Read the model definition and answer for the solid it produces. Units are mm, in the model's axes. Face numbers are marked on the shaded views. A direction names the side the tool comes from. Coordinates: 2 decimals unless noted, no trailing zeros. Write each loop counter-clockwise with the first axis right and the second up, starting at its lowest first coordinate (ties: lowest second). Pieces come first, ordered by that corner, then holes.
(1) Which of the six approach directions +Z, -Z, +X, -X, +Y, -Y give full straight-line access (tool end or side, diameter ignored) to the marked faces 4 and 5?
(2) The part is cut by section C-C, the plane z = 0. Determine the outline of the cut face in (x, y), and give its area (3 significant figures).
(3) Straight lines are drawn through the part: line 1 along Z through (x, y) = (4, -2); line 2 along Y through (x, z) = (5.5, 3); line 3 along X through (y, z) = (-7.5, 10). For each, find the intervals that lie inside material, in ascending order.
(4) Determine the mould class of the marked faces 1, 2 and 3 for opening direction Z: pulls with the +Z half, pulls with the -Z half, needs draft (parallel to the pull), parting line crosses it, or undercut.
(5) Given pin 1 (4 mm diameter, centred on x = 5, y = 11, fed in from +Z); pin 2 (2 mm diameter, centred on y = -14.5, z = 3.5, fed in from +X); pin 3 (2 mm diameter, centred on x = 4, z = 14, fed in from -Y); pin 4 (4 mm diameter, centred on y = -16, z = 0, fed in from +X), each flat-ended and moving along its own axis, determine where each tip first touches the part or whether it passes through.
(6) The part is cut by section D-D, the plane x = 20.25. Determine the outline of the cut face in (y, z).
(7) The part is cut by section A-A, the plane z = 16. Determine the outline of the cut face in (x, y).
Autodesk Inventor part; units mm, degrees
ref_plane "YZ Plane" through (0, 0, 0) normal (1, 0, 0) x (0, 1, 0)
ref_plane "XZ Plane" through (0, 0, 0) normal (0, 1, 0) x (-1, 0, 0)
ref_plane "XY Plane" through (0, 0, 0) normal (0, 0, 1) x (1, 0, 0)
sketch "Sketch_1" plane through (0, 0, 0) normal (0, 0, 1) x (1, 0, 0)
  line L0 (24, 0) -> (0, 0)
  line L1 (0, 20) -> (0, 6)
  line L2 (0, 6) -> (24, 6)
  line L3 (24, 6) -> (24, 11)
  line L4 (24, 11) -> (6, 11)
  line L5 (6, 11) -> (6, 20)
  line L6 (6, 20) -> (0, 20)
revolve "Revolution1" add sketch "Sketch_1" angle 360 about axis through (24, 0, 0) along (1, 0, 0)
sketch "Sketch2" plane through (0, 0, 0) normal (-1, 0, 0) x (0, 0, 1)
  point P0 (0, 16)
hole "Hole1" at (0, 16, 0) direction (1, 0, 0) diameter 4.5 depth 6
pattern_linear "Rectangular Pattern1" count 2 spacing 22.6274 along (0, -0.7071, 0.7071) count 2 spacing 22.6274 along (0, -0.7071, -0.7071) of "Hole1"
sketch "Sketch_4" plane through (15, 0, 0) normal (1, 0, 0) x (0, 0, -1)
  line L0 (-7.7782, -7.7782) -> (-3.5355, -3.5355)
  line L1 (-3.5355, -3.5355) -> (-2.3893, -4.6818)
  line L2 (-2.3893, -4.6818) -> (-6.364, -8.6564)
  line L3 (-6.364, -8.6564) -> (-6.364, -9.1924)
  line L4 (-6.364, -9.1924) -> (-7.7782, -7.7782)
  line L5 (-7.7782, -7.7782) -> (-3.5355, -3.5355)
revolve "Revolution2" cut sketch "Sketch_4" angle 360 about axis through (15, -7.7782, 7.7782) along (0, -0.7071, 0.7071)
thread "Thread1"
sketch "Sketch_5" plane through (15, 0, 0) normal (1, 0, 0) x (0, 0, -1)
  line L0 (-7.7782, 7.7782) -> (-3.5355, 3.5355)
  line L1 (-3.5355, 3.5355) -> (-4.6818, 2.3893)
  line L2 (-4.6818, 2.3893) -> (-8.6564, 6.364)
  line L3 (-8.6564, 6.364) -> (-9.1924, 6.364)
  line L4 (-9.1924, 6.364) -> (-7.7782, 7.7782)
  line L5 (-7.7782, 7.7782) -> (-3.5355, 3.5355)
revolve "Revolution3" cut sketch "Sketch_5" angle 360 about axis through (15, 7.7782, 7.7782) along (0, 0.7071, 0.7071)
thread "Thread2"
properties part number "STHRBN12_ss"
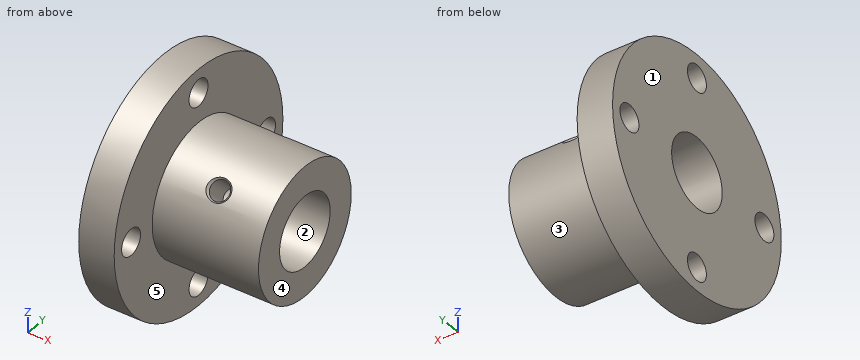
Computed:
1. face 4: +Z, -Z, +X, +Y, -Y
1. face 5: +X
2. outline: (0, -20) - (6, -20) - (6, -18.25) - (0, -18.25) - close; (0, -13.75) - (6, -13.75) - (6, -11) - (24, -11) - (24, -6) - (0, -6) - close; (0, 6) - (24, 6) - (24, 11) - (6, 11) - (6, 13.75) - (0, 13.75) - close; (0, 18.25) - (6, 18.25) - (6, 20) - (0, 20) - close
2. area: 294 mm2
3. line 1: z = -19.9 to -17.03, -14.97 to -5.66, 5.66 to 14.97, 17.03 to 19.9
3. line 2: y = -19.77 to -5.2, 5.2 to 19.77
3. line 3: x = 0 to 6
4. face 1: needs draft
4. face 2: undercut
4. face 3: parting line crosses it
5. pin 1: stops at z = 17.86
5. pin 2: stops at x = 6
5. pin 3: stops at y = -15.2
5. pin 4: passes through
6. outline: circle Ø22 at (0, 0); hole circle Ø12 at (0, 0)
7. outline: (0, -12) - (6, -12) - (6, -2.25) - (0, -2.25) - close; (0, 2.25) - (6, 2.25) - (6, 12) - (0, 12) - close
